Geometry: see drawing. Coordinates: mm, zero at the bounding-box minimum. Round coordinates to 2 decimals unless told otherwise and drop trailing zeros. Order: outer loops, then holes, each group sorted by start corner. A loop starts at its lowest first (then second) coordinate and runs counter-clockwise, first axis right, second up. Notation, with made-up numbers: (33, 77.25) -> (58, 77.25) arc R24 ccw to (58, 116.25) -> close; hole circle Ø3 at (14.25, 41.25). An arc over 180 degrees is marked (long way). Use a Markdown table: item, result.
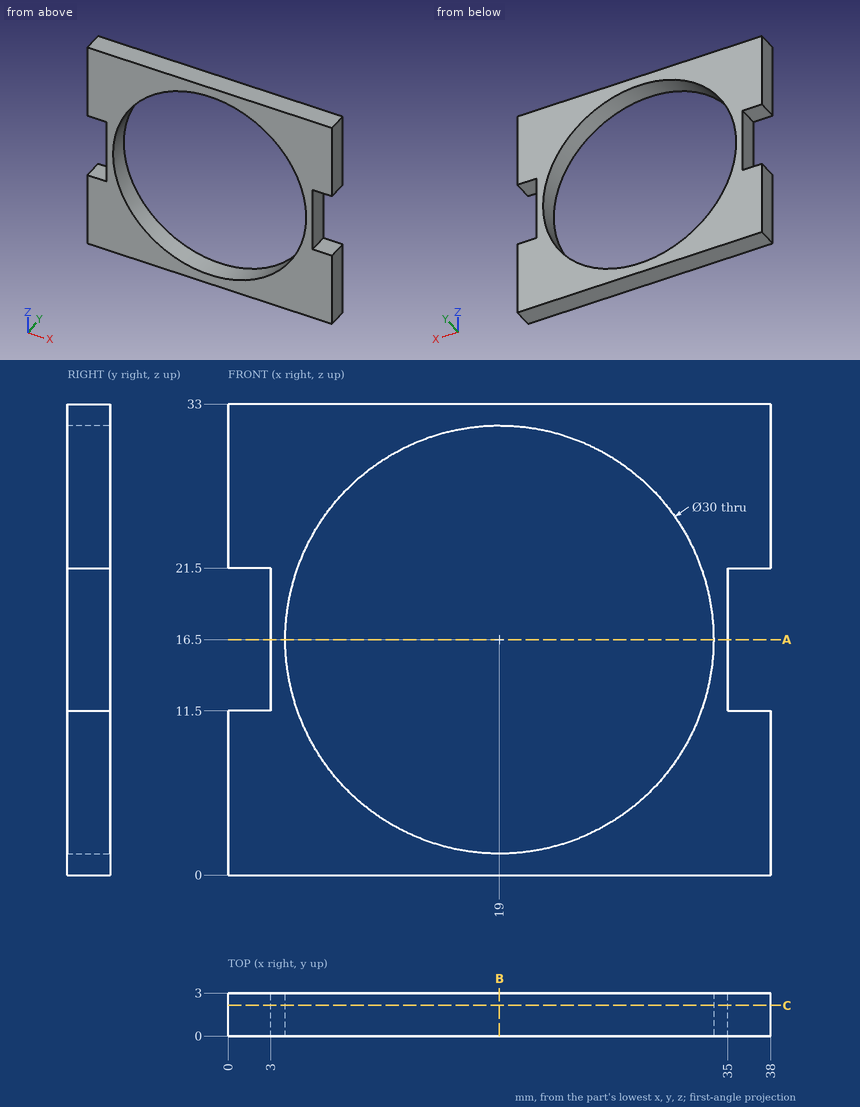
1) Cut plane C-C on y = 2.15. Return loops of the section in (x, z).
Answer key:
| item | result |
|---|---|
| outline | (0, 0) -> (38, 0) -> (38, 11.5) -> (35, 11.5) -> (35, 21.5) -> (38, 21.5) -> (38, 33) -> (0, 33) -> (0, 21.5) -> (3, 21.5) -> (3, 11.5) -> (0, 11.5) -> close; hole circle Ø30 at (19, 16.5) |
2) Cut plane A-A on z = 16.5. Return loops of the section in (x, y).
Answer key:
| item | result |
|---|---|
| outline | (3, 0) -> (4, 0) -> (4, 3) -> (3, 3) -> close; (34, 0) -> (35, 0) -> (35, 3) -> (34, 3) -> close |
3) Contact query for a flat-ended pin moving along its axis: P1, Ø0.9, axis at y = 2, z = 17.5, coming from the -X side. Output: stop coordinate, or through.
Answer key:
| item | result |
|---|---|
| P1 | stops at x = 3 |
4) Ray query, probe 1 along X at (y, z) = (0.9, 16.5); probe 2 along Z at (x, y) = (36, 1.9); probe 3 along Z at (x, y) = (19, 1.35). Return the intervals inside material, ascending.
Answer key:
| item | result |
|---|---|
| probe 1 | x = 3 to 4, 34 to 35 |
| probe 2 | z = 0 to 11.5, 21.5 to 33 |
| probe 3 | z = 0 to 1.5, 31.5 to 33 |
5) Cut plane B-B on x = 19. Return loops of the section in (y, z).
Answer key:
| item | result |
|---|---|
| outline | (0, 0) -> (3, 0) -> (3, 1.5) -> (0, 1.5) -> close; (0, 31.5) -> (3, 31.5) -> (3, 33) -> (0, 33) -> close |
